from build123d import *

# Parameters (mm, degrees)
SKETCH_1_W                  = 60
SKETCH_1_H                  = 45
SKETCH_1_R                  = 2.5
SKETCH_1_R_2                = 12
EXTRUDE_1_DEPTH             = 8
CHAMFER_1_SIZE              = 1
SKETCH_2_R                  = 4
CUT_EXTRUDE_1_DEPTH         = 6
SKETCH_3_R                  = 1.25
SKETCH_3_R_2                = 1.55
CUT_EXTRUDE_2_DEPTH         = 39.34383914
HOLE_WIZARD_2_D             = 6.2
HOLE_WIZARD_2_CSINK_D       = 13.2
HOLE_WIZARD_2_CSINK_ANGLE   = 90
HOLE_WIZARD_2_2_D           = 3.1
HOLE_WIZARD_2_2_CSINK_D     = 6.2
HOLE_WIZARD_2_2_CSINK_ANGLE = 90


with BuildPart() as part:
    # 草图1 → 凸台-拉伸1 (new body)
    with BuildSketch(Plane(origin=(0, 0, 0), x_dir=(1, 0, 0), z_dir=(0, 1, 0))):
        Rectangle(SKETCH_1_W, SKETCH_1_H)
        with Locations(Location((-20, -12.5, 0), (0, 0, 270))):
            Circle(SKETCH_1_R, mode=Mode.SUBTRACT)
        with Locations(Location((20, -12.5, 0), (0, 0, 90))):
            Circle(SKETCH_1_R, mode=Mode.SUBTRACT)
        with Locations(Location((0, -5, 0), (0, 0, 270))):
            Circle(SKETCH_1_R_2, mode=Mode.SUBTRACT)
    extrude(amount=EXTRUDE_1_DEPTH)

    # 倒角1
    chamfer_1_edges = [part.edges().sort_by_distance(p)[0] for p in [
        (0, 8, -22.5),
        (0, 0, -22.5),
    ]]
    chamfer(chamfer_1_edges, length=CHAMFER_1_SIZE)

    # 草图2 → 切除-拉伸1 (cut)
    with BuildSketch(Plane(origin=(0, 8, 0), x_dir=(1, 0, 0), z_dir=(0, 1, 0))):
        with Locations(Location((-19.5, 14.5, 0), (0, 0, 270))):
            Circle(SKETCH_2_R)
        with Locations(Location((19.5, 14.5, 0), (0, 0, 90))):
            Circle(SKETCH_2_R)
    extrude(amount=-CUT_EXTRUDE_1_DEPTH, mode=Mode.SUBTRACT)

    # 草图3 → 切除-拉伸2 (cut, through all)
    with BuildSketch(Plane(origin=(0, 0, 0), x_dir=(-1, 0, 0), z_dir=(0, -1, 0))):
        with Locations(Location((13, -18, 0), (0, 0, 90))):
            Circle(SKETCH_3_R)
        with Locations(Location((-13, -18, 0), (0, 0, 270))):
            Circle(SKETCH_3_R)
        with Locations(Location((13, 8, 0), (0, 0, 90))):
            Circle(SKETCH_3_R)
        with Locations(Location((-13, 8, 0), (0, 0, 270))):
            Circle(SKETCH_3_R)
        with Locations(Location((21, -5, 0), (0, 0, 90))):
            Circle(SKETCH_3_R_2)
        with Locations(Location((-21, -5, 0), (0, 0, 90))):
            Circle(SKETCH_3_R_2)
    extrude(amount=-CUT_EXTRUDE_2_DEPTH, mode=Mode.SUBTRACT)

    # Hole Wizard 2 (through all)
    with Locations(Plane(origin=(20, 0, 12.5), x_dir=(0, 0, -1), z_dir=(0, -1, 0))):
        with Locations((0, 0), (0, -40)):
            CounterSinkHole(HOLE_WIZARD_2_D / 2, HOLE_WIZARD_2_CSINK_D / 2, counter_sink_angle=HOLE_WIZARD_2_CSINK_ANGLE)

    # Hole Wizard 2 2 (through all)
    with Locations(Plane(origin=(-13, 8, -8), x_dir=(0, 0, 1), z_dir=(0, 1, 0))):
        with Locations((0, 0), (26, 0), (26, 26), (0, 26), (13, -8), (13, 34)):
            CounterSinkHole(HOLE_WIZARD_2_2_D / 2, HOLE_WIZARD_2_2_CSINK_D / 2, counter_sink_angle=HOLE_WIZARD_2_2_CSINK_ANGLE)


solid = part.part
The listing builds one solid part. Answer for the finished solid, in the listing's coordinates (mm). A direction names the side the tool comes from. Coordinates: 2 decimals unless noted, no trailing zeros. Write each loop counter-clockwise with the first axis right and the second up, starting at its lowest first coordinate (ties: lowest second). Pieces come first, ordered by that corner, then holes. Notation, with made-up numbers: M 74,28 L 121,28 A22 ccw 121,48 Z; hole C 10.5,25.5 d4. An arc over 180 degrees is marked long. Use one line per item in the form item = value.
Item 1: Find the intervals of material crossed by probe 1 along X at (y, z) = (4.75, -14.5); probe 2 along X at (y, z) = (4.75, 18); probe 3 along X at (y, z) = (5, 5), in increasing order.
Model answer:
probe_1 = -30 to -23.5, -15.5 to 15.5, 23.5 to 30
probe_2 = -30 to -14.55, -11.45 to 11.45, 14.55 to 30
probe_3 = -30 to -22.55, -19.45 to -12, 12 to 19.45, 22.55 to 30
Item 2: The mould has two halves that part along Z. Classify faces 1 (the face through (0, 4, 22.5)), 2 (the face through (0, 4, -22.5)), 3 (the face through (-30, 4, 0)), 4 (the face through (-16.8, 5.04, -17.45)): released by +Z, released by -Z, zero draft, split by the parting line, or undercut.
Model answer:
face_1 = released by +Z
face_2 = released by -Z
face_3 = zero draft
face_4 = undercut
Item 3: Find section A-A, the plane z = 5. Give the vertices of the cut face in (x, y).
Model answer:
outline = M -30,0 L -22.55,0 L -22.55,6.45 L -24.1,8 L -30,8 Z; M -19.45,0 L -12,0 L -12,8 L -17.9,8 L -19.45,6.45 Z; M 12,0 L 19.45,0 L 19.45,6.45 L 17.9,8 L 12,8 Z; M 22.55,0 L 30,0 L 30,8 L 24.1,8 L 22.55,6.45 Z
Item 4: Given P1, Ø10, axis at x = -20, z = 12.5, coming from the -Y side; P2, Ø4, axis at x = -13, z = 18, coming from the +Y side; P3, Ø8, axis at x = 20, z = 12.5, coming from the -Y side, each flat-ended and moving along its own axis, determine where each tip first touches the part or whether it passes through.
Model answer:
P1 = 1.6
P2 = 6.9
P3 = 2.6
Item 5: For faces 5 (the face through (20.98, 3.33, 15.62)), 6 (the face through (16.8, 5.04, -11.55)), determine the directions among +Z, -Z, +X, -X, +Y, -Y from which every point of the face is accessible in a straight line to the end or side of a thin tool.
Model answer:
face_5 = -Y
face_6 = +Y
Item 6: Find section D-D, the plane z = -14.5. Give the vertices of the cut face in (x, y).
Model answer:
outline = M -30,0 L 30,0 L 30,8 L 23.5,8 L 23.5,2 L 15.5,2 L 15.5,8 L -15.5,8 L -15.5,2 L -23.5,2 L -23.5,8 L -30,8 Z
Item 7: Find section B-B, the plane z = -8. Give the vertices of the cut face in (x, y).
Model answer:
outline = M -30,0 L -14.55,0 L -14.55,6.45 L -16.1,8 L -30,8 Z; M -11.45,0 L 11.45,0 L 11.45,6.45 L 9.9,8 L -9.9,8 L -11.45,6.45 Z; M 14.55,0 L 30,0 L 30,8 L 16.1,8 L 14.55,6.45 Z
Item 8: Find section C-C, the plane x = 0. Give the vertices of the cut face in (y, z), plus the area to 3 significant figures.
Model answer:
outline = M 0,-21.5 L 1,-22.5 L 7,-22.5 L 8,-21.5 L 8,-7 L 0,-7 Z; M 0,17 L 8,17 L 8,22.5 L 0,22.5 Z
area = 167 mm2
